The listing builds one solid part. Answer for the finished solid, in the listing's coordinates (mm). Give positions to 0.01 mm unless a question says otherwise; leave off trailing zeros. Order: outer loops, then holes, each group sorted by start corner. A loop starts at its lowest first (then second) coordinate and runs counter-clockwise, first axis right, second up. Notation, with made-up numbers: (-5, 61.25) - (38, 61.25) arc R21 cw to (38, 90.25) - close; hole circle Ø4 at (84.5, -37). An arc over 180 degrees is marked (long way). Answer as a JSON object with one key per item and string values. Group by question number.
Q1. A cutting plane is placed at B-B, the plane y = 2.25. Give the vertices of the cut face in (x, z), and give its area (3 significant figures).
Q2. Consider line 1 (X direction, y = 3.25, z = 0.05); line 2 (X direction, y = 7.25, z = -0.05); line 3 (X direction, y = 5, z = -0.1). Determine where each line is inside the solid, lowest interval first.
Q3. A cutting plane is placed at A-A, the plane y = 7.25. Give the vertices of the cut face in (x, z).
from build123d import *

# Parameters (mm, degrees)
BOSS_EXTRUDE1_DEPTH = 0.2


with BuildPart() as part:
    # Sketch1 → Boss-Extrude1 (new body, symmetric)
    with BuildSketch(Plane.XY):
        with BuildLine():
            Line((-0.32, 1.999393664), (-0.32, 4.189393664))
            ThreePointArc((-0.32, 4.189393664), (-0.378578644, 4.33081502), (-0.52, 4.389393664))
            Line((-0.52, 4.389393664), (-0.8, 4.389393664))
            ThreePointArc((-0.8, 4.389393664), (-0.941421356, 4.447972308), (-1, 4.589393664))
            Line((-1, 4.589393664), (-1, 9.979817201))
            ThreePointArc((-1, 9.979817201), (-0.87939743, 10.163382034), (-0.663039519, 10.125562961))
            add(Edge.make_bspline(
                [(-0.663039519, 10.125562961), (-0.487599251, 9.960697902), (-0.326177604, 9.738773555), (-0.310671132, 9.310865905), (-0.548453888, 9.198603212), (-0.567669208, 9.030963485)],
                knots=[0.253308427, 0.253308427, 0.253308427, 0.253308427, 0.663171976, 0.707067436, 1, 1, 1, 1], degree=3))
            Line((-0.567669208, 9.030963485), (-0.495215905, 5.324303234))
            ThreePointArc((-0.495215905, 5.324303234), (-0.483221967, 5.259888483), (-0.451053839, 5.202806733))
            add(Edge.make_bspline(
                [(-0.451053839, 5.202806733), (0, 4.642430299), (0.451053839, 5.202806733)],
                knots=[0.043404734, 0.043404734, 0.043404734, 0.956595266, 0.956595266, 0.956595266], degree=2))
            ThreePointArc((0.451053839, 5.202806733), (0.483221967, 5.259888483), (0.495215905, 5.324303234))
            Line((0.495215905, 5.324303234), (0.567669208, 9.030963485))
            add(Edge.make_bspline(
                [(0.663039519, 10.125562961), (0.487599251, 9.960697902), (0.326177604, 9.738773555), (0.310671132, 9.310865905), (0.548453888, 9.198603212), (0.567669208, 9.030963485)],
                knots=[0.253308427, 0.253308427, 0.253308427, 0.253308427, 0.663171976, 0.707067436, 1, 1, 1, 1], degree=3))
            ThreePointArc((0.663039519, 10.125562961), (0.87939743, 10.163382034), (1, 9.979817201))
            Line((1, 9.979817201), (1, 4.589393664))
            ThreePointArc((1, 4.589393664), (0.941421356, 4.447972308), (0.8, 4.389393664))
            Line((0.8, 4.389393664), (0.52, 4.389393664))
            ThreePointArc((0.52, 4.389393664), (0.378578644, 4.33081502), (0.32, 4.189393664))
            Line((0.32, 4.189393664), (0.32, 1.999393664))
            Line((0.32, 1.999393664), (0.183878151, 0.184435674))
            ThreePointArc((0.183878151, 0.184435674), (0.126073555, 0.058186541), (0, 0))
            ThreePointArc((0, 0), (-0.126073555, 0.058186541), (-0.183878151, 0.184435674))
            Line((-0.183878151, 0.184435674), (-0.32, 1.999393664))
        make_face()
    extrude(amount=BOSS_EXTRUDE1_DEPTH, both=True)

    # Esquisse1 → Enlèvement de matière-Révolution1 (revolve, cut)
    with BuildSketch(Plane.XY, mode=Mode.PRIVATE) as enl_vement_de_mati_re_r_volution1_sk:
        with BuildLine():
            Line((1, -0.500606336), (0, -0.500606336))
            Line((0, -0.500606336), (0, 0))
            ThreePointArc((0, 0), (0.121956037, 0.062291613), (0.183878151, 0.184435674))
            Line((0.183878151, 0.184435674), (0.32, 1.999393664))
            Line((0.32, 1.999393664), (1, 1.999393664))
            Line((1, 1.999393664), (1, -0.500606336))
        make_face()
    revolve(enl_vement_de_mati_re_r_volution1_sk.sketch.rotate(Axis((0, 4.922618516, 0), (0, -1, 0)), 90), axis=Axis((0, 4.922618516, 0), (0, -1, 0)), mode=Mode.SUBTRACT)  # turned: the seam where the file's is


solid = part.part
Reply:
{
 "1": {"outline": "(-0.32, -0.2) - (0.32, -0.2) - (0.32, 0.2) - (-0.32, 0.2) - close", "area": "0.256 mm^2"},
 "2": {"line 1": "x = -0.32 to 0.32", "line 2": "x = -1 to -0.53, 0.53 to 1", "line 3": "x = -1 to -0.24, 0.24 to 1"},
 "3": {"outline": "(-1, -0.2) - (-0.53, -0.2) - (-0.53, 0.2) - (-1, 0.2) - close; (0.53, -0.2) - (1, -0.2) - (1, 0.2) - (0.53, 0.2) - close"}
}
